Could you check a few things on this model? Use its own coordinates, in mm. Face numbers are marked on the shaded views. A direction names the side the tool comes from. Coordinates: 2 decimals unless noted, no trailing zeros. Write each loop counter-clockwise with the first axis right and the second up, starting at its lowest first coordinate (ties: lowest second). Pieces come first, ordered by that corner, then holes. Notation, with made-up numbers: M 28,24.5 L 72,24.5 A20 cw 72,56.5 Z; hole C -38.75,28 d4. An arc over 180 degrees is marked long. Answer as CSV lines item,"result". Start each with the question number.
Item 1: Suppose I cut it at B-B, the plane y = 26. Write out the boundary of the cut face in (x, z).
Item 2: On a 3-axis mill with a long thin cutter (end or side, diameter ignored), from which of +Z, -Z, +X, -X, +Y, -Y can I reach the whole of each face in a straight line? I mean the marked faces 4 and 5. Say none if no direction works.
Item 3: Suppose I cut it at C-C, the plane y = 4. Write out the boundary of the cut face in (x, z).
Item 4: Suppose I cut it at A-A, the plane y = 37. Write out the boundary of the cut face in (x, z), and give its area (3 significant figures).
Item 5: I'm going to push flat-ended pins straight in: P1, Ø2.5, axis at x = -5, y = 37, coming from the -Z side; P2, Ø4, axis at x = 12.5, z = -21, coming from the +Y side; P3, Ø15.5, axis at x = -2.5, y = 32, coming from the +Z side. Where does each tip first touch, or does it pass through?
Item 6: We'd pull the mould along Z, two halves only. Please class the marked faces 1, 2 and 3: +Z half, -Z half, draft (parallel to the pull), parting line (faces both ways), or undercut.
Item 7: If I drill on line 1 along Z through (x, y) = (-8, 37); line 2 along Y through (x, z) = (-5, 8.9); line 3 along Y through (x, z) = (-26, 6), over which ranges is the centre line in solid material (lowest first)? Write a range as [from, to].
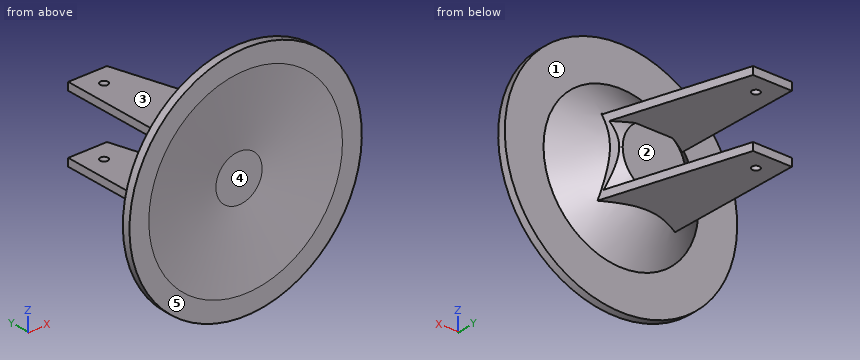
```python
from build123d import *

# Parameters (mm, degrees)
SKETCH1_R           = 30
BOSS_EXTRUDE1_DEPTH = 2
SKETCH2_R           = 20
BOSS_EXTRUDE2_DEPTH = 10
BOSS_EXTRUDE2_TAPER = 50
SKETCH3_W           = 20
SKETCH3_H           = 2
BOSS_EXTRUDE3_DEPTH = 40
CUT_EXTRUDE1_REACH  = 67.598
CUT_EXTRUDE2_REACH  = 67.598
SKETCH7_R           = 1
SKETCH8_R           = 25
CUT_EXTRUDE3_DEPTH  = 2
CUT_EXTRUDE3_DRAFT  = -84


with BuildPart() as part:
    # Sketch1 → Boss-Extrude1 (new body)
    with BuildSketch(Plane(origin=(0, 0, 0), x_dir=(1, 0, 0), z_dir=(0, 1, 0))):
        with Locations(Location((0, -0.986006094, 0), (0, 0, 270))):
            Circle(SKETCH1_R)
    extrude(amount=BOSS_EXTRUDE1_DEPTH)

    # Sketch2 → Boss-Extrude2 (add)
    with BuildSketch(Plane(origin=(0, 2, 0), x_dir=(1, 0, 0), z_dir=(0, 1, 0))):
        with Locations((0, -0.986006094)):
            Circle(SKETCH2_R)
    extrude(amount=BOSS_EXTRUDE2_DEPTH, taper=BOSS_EXTRUDE2_TAPER)

    # Sketch3 → Boss-Extrude3 (add)
    with BuildSketch(Plane(origin=(0, 2, 0), x_dir=(1, 0, 0), z_dir=(0, 1, 0))):
        with Locations((0, 8.5)):
            Rectangle(SKETCH3_W, SKETCH3_H)
        with Locations((0, -8.5)):
            Rectangle(SKETCH3_W, SKETCH3_H)
    extrude(amount=BOSS_EXTRUDE3_DEPTH)

    # Cut-Extrude1: up to this face of the body (flat: up to its plane)
    cut_extrude1_end = Plane(part.part.faces().sort_by_distance((0, 26.093864251, 9.5))[0])
    # Sketch5 → Cut-Extrude1 (cut, up to the picked face)
    with BuildSketch(Plane(origin=(0, 0, -9.5), x_dir=(-1, 0, 0), z_dir=(0, 0, -1)), mode=Mode.PRIVATE) as cut_extrude1_sk1:
        Polygon((0, 42), (-10, 6.623548306), (-10, 42), align=None)
    cut_extrude1_tool1 = split(extrude(cut_extrude1_sk1.sketch, amount=-CUT_EXTRUDE1_REACH, mode=Mode.PRIVATE), bisect_by=cut_extrude1_end, keep=Keep.BOTH, mode=Mode.PRIVATE)
    add(cut_extrude1_tool1.solids().sort_by(Axis((6.666667, 30.207849, -9.5), (0, 0, 1)))[0], mode=Mode.SUBTRACT)

    # Cut-Extrude2: up to this face of the body (flat: up to its plane)
    cut_extrude2_end = Plane(part.part.faces().sort_by_distance((-2.565960576, 24.498389602, 9.5))[0])
    # Sketch7 → Cut-Extrude2 (cut, up to the picked face)
    with BuildSketch(Plane(origin=(0, 0, -9.5), x_dir=(-1, 0, 0), z_dir=(0, 0, -1)), mode=Mode.PRIVATE) as cut_extrude2_sk1:
        with Locations((5, 37)):
            Circle(SKETCH7_R)
    cut_extrude2_tool1 = split(extrude(cut_extrude2_sk1.sketch, amount=-CUT_EXTRUDE2_REACH, mode=Mode.PRIVATE), bisect_by=cut_extrude2_end, keep=Keep.BOTH, mode=Mode.PRIVATE)
    add(cut_extrude2_tool1.solids().sort_by(Axis((-5, 37, -9.5), (0, 0, 1)))[0], mode=Mode.SUBTRACT)


with BuildPart() as cut_extrude3_tool:
    # Sketch8 → Cut-Extrude3 (with draft: the straight prism first)
    with BuildSketch(Plane.XZ):
        with Locations((0, 0.986006094)):
            Circle(SKETCH8_R)
    extrude(amount=-CUT_EXTRUDE3_DEPTH)
    # Cut-Extrude3: the draft: its side faces are tilted about the plane it starts from
    cut_extrude3_sides = [cut_extrude3_tool.faces().sort_by_distance(p)[0] for p in [
        (-25, 1, 0.986006094),
    ]]
    draft(cut_extrude3_sides, Plane.XZ, CUT_EXTRUDE3_DRAFT)


with BuildPart() as part_1:
    add(part.part)

    # Cut-Extrude3: cut by cut_extrude3_tool
    add(cut_extrude3_tool.part, mode=Mode.SUBTRACT)


solid = part_1.part
```
Ans:
1,outline,"M -10,-9.5 L 4.52,-9.5 L 4.52,-7.5 L -10,-7.5 Z; M -10,7.5 L 4.52,7.5 L 4.52,9.5 L -10,9.5 Z"
2,face 4,"-Y"
2,face 5,"+Z, -Z, +X, -X, -Y"
3,outline,"C 0,0.99 d35.23"
4,outline,"M -10,-9.5 L -6,-9.5 L -6,-7.5 L -10,-7.5 Z; M -10,7.5 L -6,7.5 L -6,9.5 L -10,9.5 Z; M -4,-9.5 L 1.41,-9.5 L 1.41,-7.5 L -4,-7.5 Z; M -4,7.5 L 1.41,7.5 L 1.41,9.5 L -4,9.5 Z"
4,area,"37.7 mm^2"
5,P1,"stops at z = -9.5"
5,P2,"stops at y = 2"
5,P3,"stops at z = 9.5"
6,face 1,"draft"
6,face 2,"undercut"
6,face 3,"+Z half"
7,line 1,"z = [-9.5, -7.5], [7.5, 9.5]"
7,line 2,"y = [1.64, 36], [38, 42]"
7,line 3,"y = [0, 2]"
